The model under review builds one solid part; all positions refer to its coordinate system, in mm. Face numbers are marked on the shaded views. A direction names the side the tool comes from. Coordinates: 2 decimals unless noted, no trailing zeros. Order: outer loops, then holes, each group sorted by start corner. A loop starts at its lowest first (then second) coordinate and runs counter-clockwise, first axis right, second up.
```python
from build123d import *

# Parameters (mm, degrees)
SKETCH_1_R          = 2
EXTRUDE_1_DEPTH     = 2
CUT_EXTRUDE_1_DEPTH = 13.952524728
SKETCH_4_W          = 2.828427125
SKETCH_4_H          = 8
EXTRUDE_2_DEPTH     = 28.28
CUT_EXTRUDE_2_DEPTH = 37.918850015
SKETCH_7_R          = 2
EXTRUDE_3_DEPTH     = 2
EXTRUDE_4_DEPTH     = 8


with BuildPart() as part:
    # 草图1 → 凸台-拉伸1 (new body)
    with BuildSketch(Plane.XY):
        with BuildLine():
            Line((3.9883881, 0), (9.9883881, 0))
            Line((9.9883881, 0), (9.9883881, 8))
            Line((9.9883881, 8), (3.9883881, 8))
            ThreePointArc((3.9883881, 8), (-0.0116119, 4), (3.9883881, 0))
        make_face()
        with Locations((3.9883881, 4)):
            Circle(SKETCH_1_R, mode=Mode.SUBTRACT)
    extrude(amount=EXTRUDE_1_DEPTH)

    # 草图2 → 切除-拉伸1 (cut, through all)
    with BuildSketch(Plane.XZ):
        Polygon((9.9883881, 2), (7.9883881, 0), (9.9883881, 0), align=None)
    extrude(amount=-CUT_EXTRUDE_1_DEPTH, mode=Mode.SUBTRACT)

    # 草图4 → 凸台-拉伸2 (add)
    with BuildSketch(Plane(origin=(3.99419405, 0, -3.99419405), x_dir=(-0.7071067811865488, 0, -0.7071067811865462), z_dir=(0.7071067811865462, 0, -0.7071067811865488))):
        with Locations((-7.062856959, 4)):
            Rectangle(SKETCH_4_W, SKETCH_4_H)
    extrude(amount=EXTRUDE_2_DEPTH)

    # 草图5 → 切除-拉伸2 (cut, through all)
    with BuildSketch(Plane(origin=(0, 8, 0), x_dir=(1, 0, 0), z_dir=(0, 1, 0))):
        Polygon((27.985367872, 19.996979772), (27.985367872, 15.996979772), (29.985367872, 17.996979772), align=None)
    extrude(amount=-CUT_EXTRUDE_2_DEPTH, mode=Mode.SUBTRACT)

    # 草图7 → 凸台-拉伸3 (add)
    with BuildSketch(Plane(origin=(0, 0, -19.998489886), x_dir=(-1, 0, 0), z_dir=(0, 0, -1))):
        with BuildLine():
            Line((-27.985367872, 8), (-33.985367872, 8))
            ThreePointArc((-33.985367872, 8), (-37.985367872, 4), (-33.985367872, 0))
            Line((-33.985367872, 0), (-27.985367872, 0))
            Line((-27.985367872, 0), (-27.985367872, 8))
        make_face()
        with Locations((-33.985367872, 4)):
            Circle(SKETCH_7_R, mode=Mode.SUBTRACT)
    extrude(amount=-EXTRUDE_3_DEPTH)

    # 草图8 → 凸台-拉伸4 (add)
    with BuildSketch(Plane(origin=(0, 8, 0), x_dir=(1, 0, 0), z_dir=(0, 1, 0))):
        Polygon((27.985367872, 15.996979772), (29.986877986, 17.998489886), (27.985367872, 17.998489886), align=None)
    extrude(amount=-EXTRUDE_4_DEPTH)


solid = part.part
```
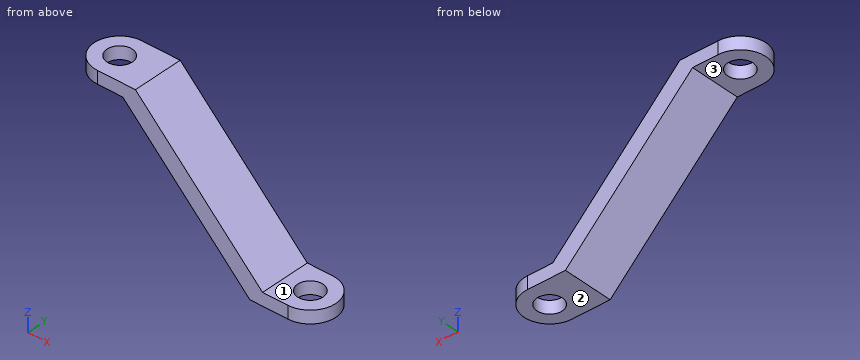
(1) We need section C-C, the plane x = 27. Write out the cut boundary in (y, z).
A:
outline: (0, -19.01) - (8, -19.01) - (8, -15.01) - (0, -15.01) - close
(2) We need section B-B, the plane z = -11. Write out the cut boundary in (x, y), and give its area (3 significant figures).
A:
outline: (18.99, 0) - (22.99, 0) - (22.99, 8) - (18.99, 8) - close
area: 32.0 mm2
(3) Machinability: for the marked faces 1, 2 and 3, which of the approach directions +Z, -Z, +X, -X, +Y, -Y give a long, thin tool a straight path to every point of the face, cutting with its end or side? Answer none if there is none.
A:
face 1: +Z, +X, +Y, -Y
face 2: -Z, +X, -X, +Y, -Y
face 3: -Z, -X, +Y, -Y
(4) For pin 1 Ø4 at (x, y) = (5, 4) entering from -Z; pin 2 Ø2 at (y, z) = (6, -12.5) entering from +X; pin 3 Ø1 at (y, z) = (3.5, -12.5) entering from +X, all flat-tipped, find the tip position at first contact; note any pin that passes through.
A:
pin 1: stops at z = 0
pin 2: stops at x = 25.49
pin 3: stops at x = 24.99
(5) We need section A-A, the plane y = 4. Count the separate pieces of the cut face and the enclosed holes in it, and give its area (4 significant figures).
A:
separate pieces: 3
enclosed holes: 0
area: 100.0 mm2
(6) Wall thickness on probe 1 along Z at (x, y) = (2.5, 7.5); probe 2 along Z at (x, y) = (30, 2.25); probe 3 along X at (y, z) = (6, -10.25): over which ranges is each line inside the solid? List them lowest first.
A:
probe 1: z = 0 to 2
probe 2: z = -20 to -18
probe 3: x = 18.24 to 22.24
